For this review, use the dimensioned drawing (mm, ordinates from the lowest corner) and the shaded views. A direction names the side the tool comes from. Coordinates: 2 decimals unless noted, no trailing zeros. Loops run counter-clockwise (first coordinate to the right, second up) from the corner with the lowest first, then second, coordinate; pieces in that order, holes last. Notation, with made-up numbers: (-14, -20) - (-9, -20) arc R23 ccw to (-9, -7) - close; hole circle Ø2 at (63, -4.75). An arc over 180 degrees is marked (long way). Answer in a Markdown table with one row per item. Add a question column.
(1) To check wall thickness, follow L1, parallel to Z at x = 7.75, y = 7.5 (1 decimal); L2, parallel to Z at x = 19.25, y = 11.5 (1 decimal); L3, parallel to Z at x = 7, y = 11.75 (1 decimal). State the ranges of each line that lie inside material, in increasing order. Write a range as [from, to].
(2) We need section B-B, the plane x = 7.75. Write out the cut boundary in (y, z) (1 decimal).
(3) We need section A-A, the plane z = 5.25. Write out the cut boundary in (x, y) (1 decimal), plus the area to 3 significant figures.
(4) The part is to be moulded in two halves that separate along Z. For the marked faces 3, 4, 5 and 6, say which applies: released by +Z, released by -Z, zero draft, split by the parting line, or undercut.
(5) Clearance check with flat-ended pins moving along their axes: pin 1 (1.5 mm diameter, centred on y = 3, z = 16, fed in from +X); pin 2 (1 mm diameter, centred on x = 2.5, y = 2, fed in from -Z); pin 3 (1 mm diameter, centred on y = 3, z = 13, fed in from +X); pin 4 (2.5 mm diameter, centred on x = 14.72, z = 4.55, fed in from +Y). State where each tip first meets the part, or that it passes through.
(6) We need section C-C, the plane y = 11.5. Give the number of separate pieces and of enclosed holes in the cut face, plus the area to 3 significant figures.
(7) We need section D-D, the plane z = 12.5. Write out the cut boundary in (x, y) (1 decimal).
(8) For the marked faces 1 and 2, list the 3-axis set-ups (+Z, -Z, +X, -X, +Y, -Y) from which the entire face can be reached by the end or side of a thin tool; tool diameter is ignored.
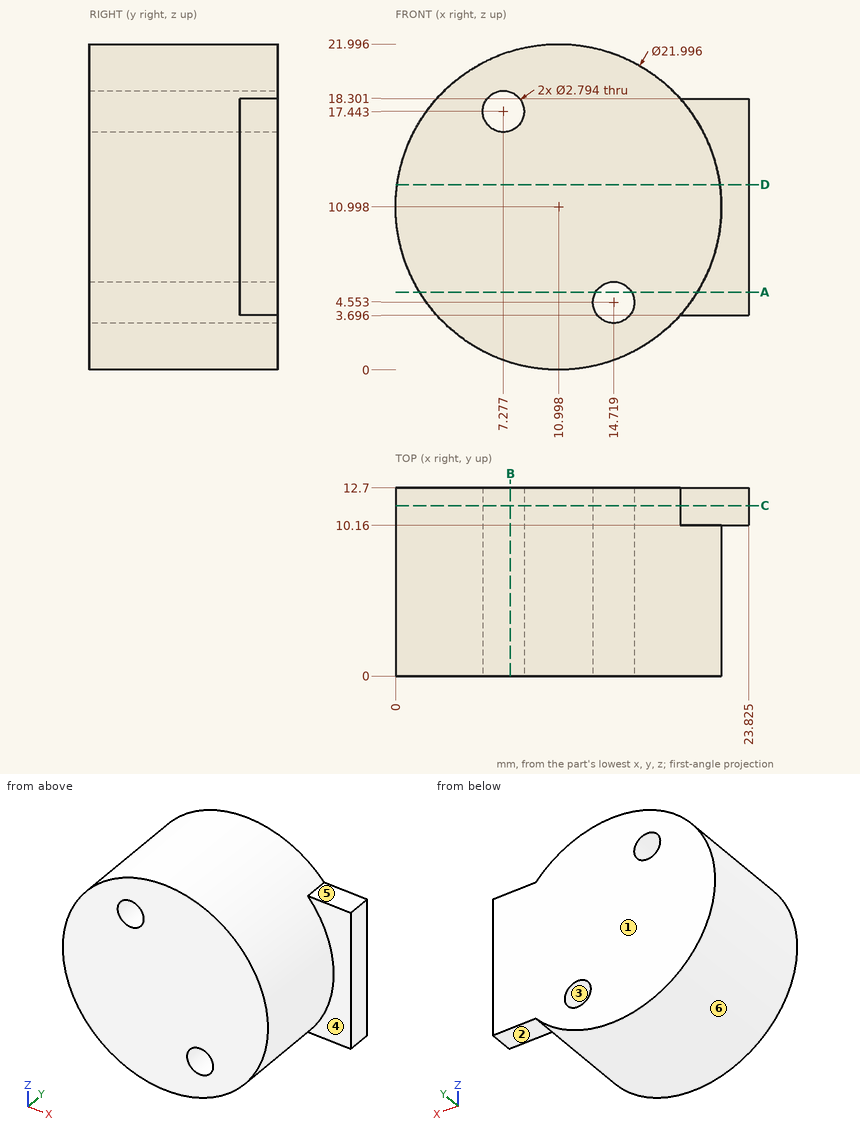
Responses:
| question | item | result |
|---|---|---|
| 1 | L1 | z = [0.5, 16.1], [18.8, 21.5] |
| 1 | L2 | z = [3.7, 18.3] |
| 1 | L3 | z = [0.8, 16.1], [18.8, 21.2] |
| 2 | outline | (0, 0.5) - (12.7, 0.5) - (12.7, 16.1) - (0, 16.1) - close; (0, 18.8) - (12.7, 18.8) - (12.7, 21.5) - (0, 21.5) - close |
| 3 | outline | (1.6, 0) - (13.5, 0) - (13.5, 12.7) - (1.6, 12.7) - close; (15.9, 0) - (20.4, 0) - (20.4, 10.2) - (23.8, 10.2) - (23.8, 12.7) - (15.9, 12.7) - close |
| 3 | area | 216 mm2 |
| 4 | face 3 | undercut |
| 4 | face 4 | zero draft |
| 4 | face 5 | released by +Z |
| 4 | face 6 | split by the parting line |
| 5 | pin 1 | stops at x = 21.14 |
| 5 | pin 2 | stops at z = 3.45 |
| 5 | pin 3 | stops at x = 21.89 |
| 5 | pin 4 | passes through |
| 6 | separate pieces | 1 |
| 6 | enclosed holes | 2 |
| 6 | area | 407 mm2 |
| 7 | outline | (0.1, 0) - (21.9, 0) - (21.9, 10.2) - (23.8, 10.2) - (23.8, 12.7) - (0.1, 12.7) - close |
| 8 | face 1 | +Z, -Z, +X, -X, +Y |
| 8 | face 2 | -Z, +X, +Y, -Y |
